Read the model definition and answer for the solid it produces. Units are mm, in the model's axes. Coordinates: 2 decimals unless noted, no trailing zeros. Loops run counter-clockwise (first coordinate to the right, second up) from the corner with the lowest first, then second, coordinate; pieces in that order, holes last. Notation, with made-up numbers: M 73.5,74.5 L 115.5,74.5 A15 ccw 115.5,95.5 Z; hole C 84.25,-38 d9. An arc over 180 degrees is marked long. Use one line per item in the form item = value. Start each with the question number.
1. The part is cut by section D-D (z = 93). Give the vertices of the cut face in (x, y), plus the area to 3 significant figures.
2. Flat-ended cylindrical pins translate along their axes: pin 1 (1 mm diameter, centred on x = 4, y = -45, fed in from +Z); pin 2 (3 mm diameter, centred on x = 24, y = -41.5, fed in from +Z); pin 3 (9 mm diameter, centred on y = -89.5, z = 140.5, fed in from +X); pin 4 (2 mm diameter, centred on x = 23, z = 100, fed in from +Y). Find the tip coordinate at first contact, or state that the pin passes through.
3. The part is cut by section C-C (y = -87.5). Give the number of separate pieces and of enclosed holes in the cut face, plus the area to 3 significant figures.
4. Find the intervals of material crossed by probe 1 along Z at (x, y) = (42.5, -10); probe 2 along Z at (x, y) = (9, -87); probe 3 along Z at (x, y) = (-39.5, -92.5), in increasing order. Write a range as [from, to].
5. For a pull along Z with two mould halves and no side action, classify faces 1 (the flat face through (1, -71, 0)), 2 (the flat face through (-63.5, -71, 54)), 3 (the flat face through (1, -69, 88.9)), 4 (the flat face through (0.89, -90.65, 137.8)) as released by +Z, released by -Z, zero draft, split by the parting line, or undercut.
6. The part is cut by section B-B (y = -61.5). Give the vertices of the cut face in (x, z).
7. The part is cut by section A-A (x = 4). Give the vertices of the cut face in (y, z).
from build123d import *

# Parameters (mm, degrees)
F1_DEPTH = 63.5
F2_W     = 15.875
F2_H     = 15.875
F3_DEPTH = 0.4064


# Not quite as in the source:
# - the dataset's text gives a spline's control points without its knots; the knots are read off the source's solid


with BuildPart() as f1:
    # F0 (on Right) → F1 (new body, symmetric)
    with BuildSketch(Plane.YZ):
        Polygon((-139.7, 0), (0, 0), (0, 88.9), (-139.2936, 88.9), (-139.2936, 89.154), (-40.6298144724, 187.8177855276), (-40.9171826682, 188.1051537235), (-139.7, 89.3223363917), align=None)
    extrude(amount=F1_DEPTH, both=True)

    # F2 (on face) → F3 (cut, through all)
    with BuildSketch(Plane(origin=(0, -114.5111681959, 114.5111681959), x_dir=(1, 0, 0), z_dir=(0, -0.7071067812, 0.7071067812))):
        with Locations((25.435084784, 38.0925593219)):
            Rectangle(F2_W, F2_H)
        with BuildLine():
            add(Edge.make_bspline(
                [(-19.471708816, 43.9859181219), (-21.014403216, 45.5287903219), (-23.182750416, 46.4269343219), (-25.364915216, 46.4269343219)],
                knots=[7, 7, 7, 7, 8, 8, 8, 8], degree=3))
            add(Edge.make_bspline(
                [(-25.364915216, 46.4269343219), (-27.546648216, 46.4269343219), (-29.715351016, 45.5287903219), (-31.258045416, 43.9859181219)],
                knots=[0, 0, 0, 0, 1, 1, 1, 1], degree=3))
            add(Edge.make_bspline(
                [(-31.258045416, 43.9859181219), (-32.800790616, 42.4430205219), (-33.699290216, 40.2745209219), (-33.699290216, 38.0925593219), (-33.699290216, 35.9107755219), (-32.800790616, 33.7420981219), (-31.258045416, 32.1993529219)],
                knots=[1, 1, 1, 1, 2, 2, 2, 3, 3, 3, 3], degree=3))
            add(Edge.make_bspline(
                [(-31.258045416, 32.1993529219), (-29.715351016, 30.6563029219), (-27.546648216, 29.7581843219), (-25.364915216, 29.7581843219), (-23.182750416, 29.7581843219), (-21.014403216, 30.6563029219), (-19.471708816, 32.1993529219)],
                knots=[3, 3, 3, 3, 4, 4, 4, 5, 5, 5, 5], degree=3))
            add(Edge.make_bspline(
                [(-19.471708816, 32.1993529219), (-17.928658816, 33.7420981219), (-17.030540216, 35.9107755219), (-17.030540216, 38.0925593219), (-17.030540216, 40.2745209219), (-17.928658816, 42.4430205219), (-19.471708816, 43.9859181219)],
                knots=[5, 5, 5, 5, 6, 6, 6, 7, 7, 7, 7], degree=3))
        make_face()
    extrude(amount=-F3_DEPTH, mode=Mode.SUBTRACT)


solid = f1.part
Computed values:
q1.outline = M -63.5,-136.02 L 63.5,-136.02 L 63.5,-135.45 L -63.5,-135.45 Z
q1.area = 73.0 mm²
q2.pin_1 = 184.52
q2.pin_2 = 188.11
q2.pin_3 = 63.5
q2.pin_4 = -127.45
q3.separate_pieces = 4
q3.enclosed_holes = 0
q3.area = 11,300 mm²
q4.probe_1 = [0, 88.9]
q4.probe_2 = [0, 88.9], [141.45, 142.02]
q4.probe_3 = [0, 88.9], [135.95, 136.52]
q5.face_1 = released by -Z
q5.face_2 = zero draft
q5.face_3 = undercut
q5.face_4 = undercut
q6.outline = M -63.5,0 L 63.5,0 L 63.5,88.9 L -63.5,88.9 Z; M -63.5,166.95 L 63.5,166.95 L 63.5,167.52 L -63.5,167.52 Z
q7.outline = M -139.7,0 L 0,0 L 0,88.9 L -139.29,88.9 L -139.29,89.15 L -40.63,187.82 L -40.92,188.11 L -139.7,89.32 Z
